Drawing for the job (mm, zero at the part's lowest x, y, z). Give positions to 0.01 mm unless a question says otherwise; leave off trailing zeros. Order: outer loops, then holes, each group sorted by start corner. A loop starts at its lowest first (then second) coordinate and runs counter-clockwise, first axis right, second up. Notation, with made-up numbers: (11, 71.25) - (68, 71.25) arc R31 cw to (68, 103.25) - close; hole circle Ø10 at (62.5, 30.25). An arc over 180 degrees is marked (long way). Use a Markdown table: item, result. Add a question column.
(1) Slice it at C-C (y = 34). Write the cut outline in (x, z), then the cut area to 3 significant figures.
(2) Slice it at B-B (x = 135). Write the cut outline in (y, z).
(3) Mould opens along Z. For the marked faces 1, 2, 3 and 4 say: +Z half, -Z half, draft (parallel to the pull), parting line (faces both ways), or undercut.
(4) Slice it at D-D (x = 80). Write the cut outline in (y, z).
(5) Flat gauge pins, fed straight in: pin 1 (13 mm diameter, centred on x = 187.31, z = 152, fed in from -Y); pin 2 (23 mm diameter, centred on x = 167.33, z = 90.5, fed in from +Y); pin 3 (5 mm diameter, centred on x = 236.5, z = 44, fed in from +Y); pin 4 (16.5 mm diameter, centred on x = 102.67, z = 90.5, fed in from -Y). Where does each tip first touch, or does it go through?
(6) Slice it at A-A (z = 135). Write the cut outline in (x, y), then the cut area to 4 significant figures.
(7) Wall check: line 1 (Z direction, x = 135, y = 38.5); line 2 (Z direction, x = 137.5, y = 5.5); line 3 (Y direction, x = 18, z = 94.5). Give the ranges that are in metal, low to high.
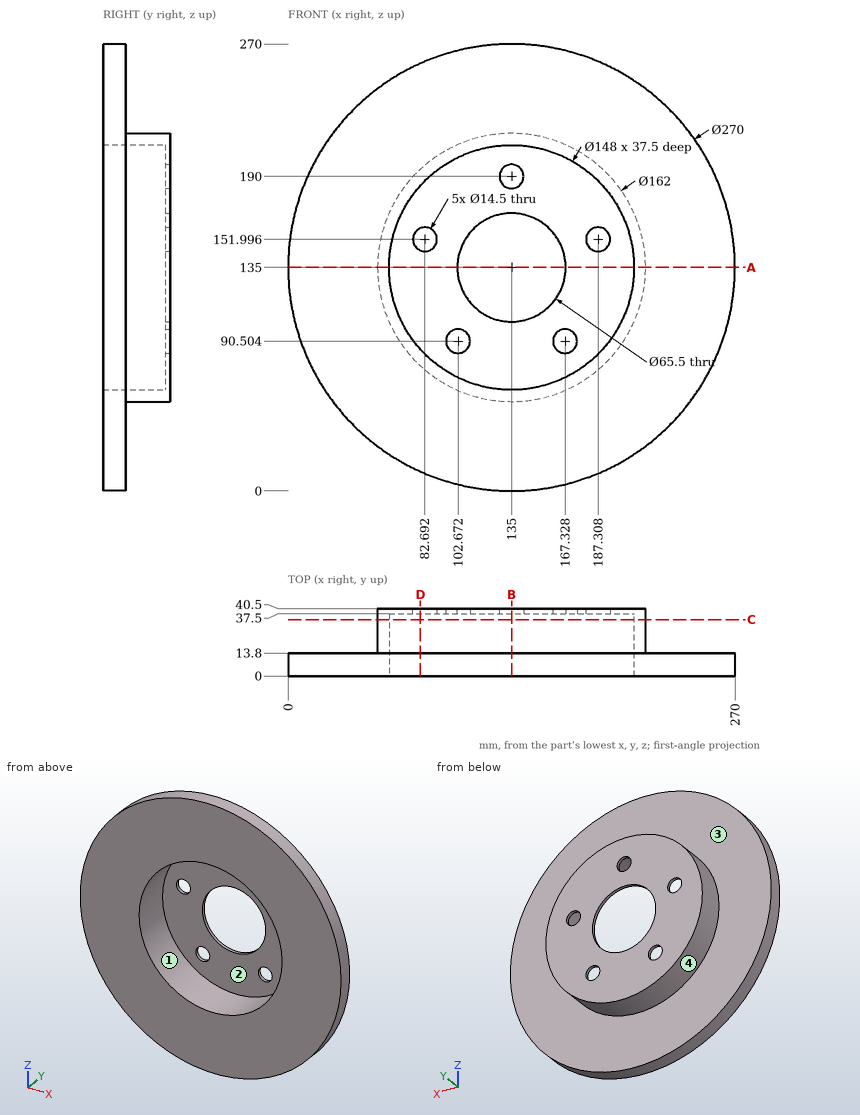
Solution:
| question | item | result |
|---|---|---|
| 1 | outline | circle Ø162 at (135, 135); hole circle Ø148 at (135, 135) |
| 1 | area | 3,410 mm2 |
| 2 | outline | (0, 0) - (13.8, 0) - (13.8, 54) - (40.5, 54) - (40.5, 102.25) - (37.5, 102.25) - (37.5, 61) - (0, 61) - close; (0, 209) - (37.5, 209) - (37.5, 197.25) - (40.5, 197.25) - (40.5, 216) - (13.8, 216) - (13.8, 270) - (0, 270) - close; (37.5, 167.75) - (40.5, 167.75) - (40.5, 182.75) - (37.5, 182.75) - close |
| 3 | face 1 | undercut |
| 3 | face 2 | undercut |
| 3 | face 3 | draft |
| 3 | face 4 | parting line |
| 4 | outline | (0, 11.71) - (13.8, 11.71) - (13.8, 75.54) - (40.5, 75.54) - (40.5, 145.26) - (37.5, 145.26) - (37.5, 85.49) - (0, 85.49) - close; (0, 184.51) - (37.5, 184.51) - (37.5, 158.73) - (40.5, 158.73) - (40.5, 194.46) - (13.8, 194.46) - (13.8, 258.29) - (0, 258.29) - close |
| 5 | pin 1 | through |
| 5 | pin 2 | y = 40.5 |
| 5 | pin 3 | y = 13.8 |
| 5 | pin 4 | y = 37.5 |
| 6 | outline | (0, 0) - (61, 0) - (61, 37.5) - (102.25, 37.5) - (102.25, 40.5) - (54, 40.5) - (54, 13.8) - (0, 13.8) - close; (167.75, 37.5) - (209, 37.5) - (209, 0) - (270, 0) - (270, 13.8) - (216, 13.8) - (216, 40.5) - (167.75, 40.5) - close |
| 6 | area | 2,305 mm2 |
| 7 | line 1 | 54 to 102.25, 167.75 to 182.75, 197.25 to 216 |
| 7 | line 2 | 0.02 to 61.04, 208.96 to 269.98 |
| 7 | line 3 | 0 to 13.8 |
